```python
from build123d import *

# Parameters (mm, degrees)
F0_R     = 20.5
F1_DEPTH = 2
F2_R     = 19
F3_DEPTH = 20
F4_D     = 21
F5_SIZE  = 1
F6_SIZE  = 3


with BuildPart() as f1:
    # F0 (on Top) → F1 (new body)
    with BuildSketch(Plane.XY):
        Circle(F0_R)
    extrude(amount=F1_DEPTH)

    # F2 (on face) → F3 (join)
    with BuildSketch(Plane.XY.offset(2)):
        Circle(F2_R)
    extrude(amount=F3_DEPTH)

    # F4 (through all)
    with Locations(Plane(origin=(0, 0, 0), x_dir=(1, 0, 0), z_dir=(0, 0, -1))):
        with Locations((0, 0)):
            Hole(F4_D / 2)

    # F5
    f5_edges = [f1.edges().sort_by_distance(p)[0] for p in [
        (-20.5, 0, 0),
        (-10.5, 0, 0),
        (-10.5, 0, 22),
    ]]
    chamfer(f5_edges, length=F5_SIZE)

    # F6
    f6_edges = [f1.edges().sort_by_distance(p)[0] for p in [
        (-19, 0, 22),
    ]]
    chamfer(f6_edges, length=F6_SIZE)


solid = f1.part
```
Geometry: final body of the model. Coordinates: model frame, mm. A direction names the side the tool comes from. Coordinates: 2 decimals unless noted, no trailing zeros. Order: outer loops, then holes, each group sorted by start corner. A loop starts at its lowest first (then second) coordinate and runs counter-clockwise, first axis right, second up. Notation, with made-up numbers: (16.5, 39) - (47.5, 39) arc R26 ccw to (47.5, 54) - close; hole circle Ø11 at (21, 58). An arc over 180 degrees is marked (long way). Return JSON: item names as keys, results as strings. Group by question number.
1. Cut plane A-A (y = 0). Output: boundary loops of the cut face in (x, z).
2. Cut plane C-C (z = 12.25). Output: boundary loops of the cut face in (x, y), plus the area to 3 significant figures.
3. Set-up query: faces 4 (the face through (14, -14, 2)), 5 (the face through (8.4, -8.4, 0)). Return all of +Z, -Z, +X, -X, +Y, -Y with unobstructed straight access to the full face (end or side cutting, diameter ignored); none if empty.
4. Pin query (flat end, axial travel): pin 1 (24 mm diameter, centred on x = 0, y = 0, fed in from +Z); pin 2 (1.5 mm diameter, centred on x = 8, y = 2, fed in from +Z); pin 3 (2 mm diameter, centred on y = -15, z = 14, fed in from -X); pin 4 (5 mm diameter, centred on x = -14.5, z = 18, fed in from +Y). Return the tip coordinate at first contact, or that it passes through.
5. Pull-direction query (Y, two-part tool) for faces 1 (the face through (-10, -3.2, 11.1)), 2 (the face through (-11, 4, 22)), 3 (the face through (8.767, -16.856, 10.381)); classes: pulls with the +Y half, pulls with the -Y half, needs draft (parallel to the pull), parting line crosses it, or undercut.
6. Material intervals for line 1 along Y through (x, z) = (0, 11); line 2 along X through (y, z) = (6.5, 1.75); line 3 along X through (y, z) = (-2, 17.5), sorted ascending. Write a range as [from, to].
Resolved:
{
 "1": {"outline": "(-20.5, 1) - (-19.5, 0) - (-11.5, 0) - (-10.5, 1) - (-10.5, 21) - (-11.5, 22) - (-16, 22) - (-19, 19) - (-19, 2) - (-20.5, 2) - close; (10.5, 1) - (11.5, 0) - (19.5, 0) - (20.5, 1) - (20.5, 2) - (19, 2) - (19, 19) - (16, 22) - (11.5, 22) - (10.5, 21) - close"},
 "2": {"outline": "circle Ø38 at (0, 0); hole circle Ø21 at (0, 0)", "area": "788 mm²"},
 "3": {"face 4": "+Z", "face 5": "-Z, +X, -X, +Y, -Y"},
 "4": {"pin 1": "stops at z = 22", "pin 2": "passes through", "pin 3": "stops at x = -12.85", "pin 4": "stops at y = 14.73"},
 "5": {"face 1": "undercut", "face 2": "needs draft", "face 3": "parting line crosses it"},
 "6": {"line 1": "y = [-19, -10.5], [10.5, 19]", "line 2": "x = [-19.44, -8.25], [8.25, 19.44]", "line 3": "x = [-18.89, -10.31], [10.31, 18.89]"}
}
